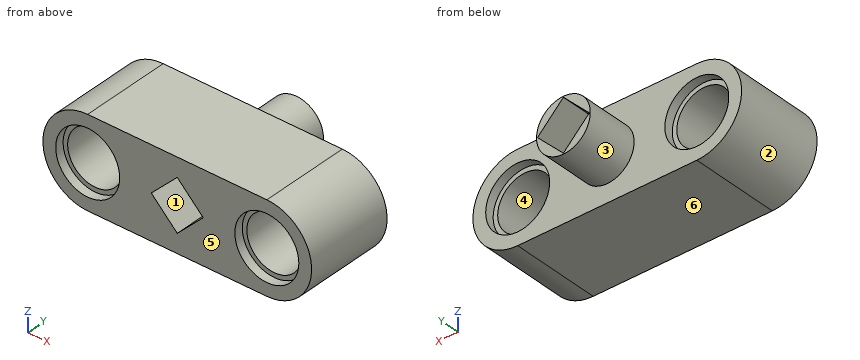
Autodesk Inventor part; units mm, degrees
ref_plane "YZ Plane" through (0, 0, 0) normal (1, 0, 0) x (0, 1, 0)
ref_plane "XZ Plane" through (0, 0, 0) normal (0, 1, 0) x (-1, 0, 0)
ref_plane "XY Plane" through (0, 0, 0) normal (0, 0, 1) x (1, 0, 0)
sketch "Sketch1" plane through (0, 0, 0) normal (0, 1, 0) x (-1, 0, 0)
  line L0 (-8.001, 0) -> (8.001, 0) construction
  line L1 (-8.001, -4.0005) -> (8.001, -4.0005)
  line L2 (8.001, 4.0005) -> (-8.001, 4.0005)
  arc A0 (-8.001, 4.0005) -> (-8.001, -4.0005) centre (-8.001, 0) ccw
  arc A1 (8.001, -4.0005) -> (8.001, 4.0005) centre (8.001, 0) ccw
  line L3 (-2.3169, 0) -> (0, 2.3169)
  line L4 (0, 2.3169) -> (2.3169, 0)
  line L5 (2.3169, 0) -> (0, -2.3169)
  line L6 (0, -2.3169) -> (-2.3169, 0)
  line L7 (-2.3169, 0) -> (2.3169, 0) construction
  line L8 (0, 2.3169) -> (0, -2.3169) construction
  point P0 (0, 0)
  dimension "d0" = 8.001
  dimension "d1" = 8.001
  dimension "d2" = 3.2766
  dimension "d3" = 3.2766
extrude "Extrusion1" add sketch "Sketch1" along normal blind 8.001
sketch "Sketch2" plane through (0, 8.001, 0) normal (0, 1, 0) x (1, 0, 0)
  circle A0 centre (-8.001, 0) radius 2.8575
  point P0 (0, 0)
  dimension "d6" = 8.001
  dimension "d7" = 5.715
extrude "Extrusion2" cut sketch "Sketch2" against normal blind 0.7874
sketch "Sketch3" plane through (0, 8.001, 0) normal (0, 1, 0) x (1, 0, 0)
  circle A0 centre (8.001, 0) radius 2.8575
  point P0 (0, 0)
  dimension "d10" = 8.001
  dimension "d11" = 5.715
extrude "Extrusion3" cut sketch "Sketch3" against normal blind 0.7874
sketch "Sketch4" plane through (0, 0, 0) normal (0, -1, 0) x (1, 0, 0)
  circle A0 centre (8.001, 0) radius 2.8575
  circle A1 centre (8.001, 0) radius 2.8575
  point P0 (0, 0)
extrude "Extrusion4" cut sketch "Sketch4" against normal blind 0.7874
sketch "Sketch5" plane through (0, 0, 0) normal (0, -1, 0) x (1, 0, 0)
  circle A0 centre (-8.001, 0) radius 2.8575
  circle A1 centre (-8.001, 0) radius 2.8575
  point P0 (0, 0)
extrude "Extrusion5" cut sketch "Sketch5" against normal blind 0.7874
sketch "Sketch6" plane through (-8.001, 7.2136, 0) normal (0, 1, 0) x (1, 0, 0)
  circle A0 centre (0, 0) radius 2.4511
  point P0 (8.001, 0)
  dimension "d18" = 4.9022
extrude "Extrusion6" cut sketch "Sketch6" against normal through all
sketch "Sketch7" plane through (8.001, 7.2136, 0) normal (0, 1, 0) x (1, 0, 0)
  circle A0 centre (0, 0) radius 2.4511
  point P0 (-8.001, 0)
  dimension "d21" = 4.9022
extrude "Extrusion7" cut sketch "Sketch7" against normal through all
sketch "Sketch8" plane through (0, 8.001, 0) normal (0, 1, 0) x (1, 0, 0)
  circle A0 centre (0, 0) radius 2.4003
  dimension "d24" = 4.8006
extrude "Extrusion8" add sketch "Sketch8" along normal blind 4.6482
sketch "Sketch9" plane through (0, 12.6492, 0) normal (0, 1, 0) x (1, 0, 0)
  line L0 (2.3169, 0) -> (0, 2.3169)
  line L1 (0, 2.3169) -> (-2.3169, 0)
  line L2 (-2.3169, 0) -> (0, -2.3169)
  line L3 (0, -2.3169) -> (2.3169, 0)
  circle A0 centre (0, 0) radius 2.4003
  line L4 (-1.6383, -1.6383) -> (1.6383, 1.6383) construction
  line L5 (1.6383, -1.6383) -> (-1.6383, 1.6383) construction
  dimension "d27" = 3.2766
  dimension "d28" = 3.2766
extrude "Extrusion9" cut sketch "Sketch9" against normal blind 4.6482 contours L3 L2 L1 L0
properties part number "VexLegoCoupler"
Here's how the part is built. I have some questions about the finished solid (model axes, mm). Face numbers are marked on the shaded views. A direction names the side the tool comes from. Round coordinates to 2 decimals unless told otherwise and drop trailing zeros. Order: outer loops, then holes, each group sorted by start corner. A loop starts at its lowest first (then second) coordinate and runs counter-clockwise, first axis right, second up. Notation, with made-up numbers: M -11.75,1 L 34.25,1 A11 cw 34.25,11 Z; hole C -9,77 d6. An arc over 180 degrees is marked long. Return JSON: item names as keys, results as strings. Group by question number.
1. On a 3-axis mill with a long thin cutter (end or side, diameter ignored), from which of +Z, -Z, +X, -X, +Y, -Y can I reach the whole of each face in a straight line? I mean the marked faces 1, 2 and 3. Say none if no direction works.
2. If we section it at B-B on x = -6: List the corners of the cut face in (y, z) for me.
3. If we section it at D-D on z = 0.5: State how many separate pieces and enclosed holes the cut face has, then the cut area to 3 significant figures.
4. If we section it at C-C on y = 12: List the corners of the cut face in (x, z) for me, then the cut area to 3 significant figures.
5. Please list where these lines run through material, in increasing order: probe 1 along Y at (x, z) = (-10, 3); probe 2 along X at (y, z) = (11.5, -0.25); probe 3 along Z at (x, y) = (0.75, 11.5).
6. If we section it at A-A on y = 6.25: List the corners of the cut face in (x, z) for me.
7. I'm going to push flat-ended pins straight in: pin 1 Ø4.5 at (x, z) = (8.001, 0) entering from +Y; pin 2 Ø4 at (x, z) = (-6, 1.5) entering from +Y; pin 3 Ø3 at (x, z) = (7.5, -1) entering from +Y; pin 4 Ø3 at (y, z) = (8, 3) entering from +X. Where does each tip first touch, or does it pass through?
8. If we mould it in two halves opening along Z, with no side actions, what happens to the marked faces 4, 5 and 6? For each: pulls with the +Z half, pulls with the -Z half, needs draft (parallel to the pull), parting line crosses it, or undercut.
Reply:
{
 "1": {"face 1": "+Y, -Y", "face 2": "-X, +Y, -Y", "face 3": "+Y"},
 "2": {"outline": "M 0,-4 L 8,-4 L 8,-2.04 L 7.21,-2.04 L 7.21,-1.42 L 0.79,-1.42 L 0.79,-2.04 L 0,-2.04 Z; M 0,2.04 L 0.79,2.04 L 0.79,1.42 L 7.21,1.42 L 7.21,2.04 L 8,2.04 L 8,4 L 0,4 Z"},
 "3": {"separate pieces": "4", "enclosed holes": "0", "area": "88.0 mm^2"},
 "4": {"outline": "C 0,0 d4.8; hole M -2.32,0 L 0,-2.32 L 2.32,0 L 0,2.32 Z", "area": "7.36 mm^2"},
 "5": {"probe 1": "0 to 8", "probe 2": "-2.39 to -2.07, 2.07 to 2.39", "probe 3": "-2.28 to -1.57, 1.57 to 2.28"},
 "6": {"outline": "M -8,-4 L 8,-4 A4 ccw 8,4 L -8,4 A4 ccw Z; hole C -8,0 d4.9; hole M -2.32,0 L 0,-2.32 L 2.32,0 L 0,2.32 Z; hole C 8,0 d4.9"},
 "7": {"pin 1": "through", "pin 2": "y = 8", "pin 3": "y = 7.21", "pin 4": "x = 11.71"},
 "8": {"face 4": "undercut", "face 5": "needs draft", "face 6": "pulls with the -Z half"}
}
